Source: CAD feature listing. Evaluate the final solid. Frame: model axes, mm. Round coordinates to 2 decimals unless told otherwise and drop trailing zeros. Loops run counter-clockwise (first coordinate to the right, second up) from the corner with the lowest first, then second, coordinate; pieces in that order, holes last. Notation, with made-up numbers: M 41,27.5 L 73,27.5 A11 ccw 73,31.5 Z; hole C -1,73 d9. An arc over 180 degrees is marked long. One line per item, written item: value.
from build123d import *

# Parameters (mm, degrees)
SKETCH1_W                = 270
SKETCH1_H                = 25
BOSS_EXTRUDE1_DEPTH      = 4
M5_CLEARANCE_SLOT1_DEPTH = 4
LPATTERN1_COUNT          = 4
LPATTERN1_PITCH          = 82
M3_TAPPED_HOLE1_D        = 2.5
LPATTERN2_COUNT          = 8
LPATTERN2_PITCH          = 35.714285714
CHAMFER1_SIZE            = 2
M5_TAPPED_HOLE1_D        = 4.2


# Read off the part's stored shape, not the designer's step: M5 Clearance Slot1
with BuildPart() as part:
    # Sketch1 → Boss-Extrude1 (new body)
    with BuildSketch(Plane.XY):
        Rectangle(SKETCH1_W, SKETCH1_H)
    extrude(amount=BOSS_EXTRUDE1_DEPTH)

    # M5 Clearance Slot1 outline → M5 Clearance Slot1 (cut)
    with BuildSketch(Plane.XY):
        with BuildLine():
            Line((-120.25, 2.25), (-120.25, 6.75))
            ThreePointArc((-120.25, 6.75), (-123, 9.5), (-125.75, 6.75))
            Line((-125.75, 6.75), (-125.75, 2.25))
            ThreePointArc((-125.75, 2.25), (-123, -0.5), (-120.25, 2.25))
        make_face()
    m5_clearance_slot1 = extrude(amount=M5_CLEARANCE_SLOT1_DEPTH, mode=Mode.SUBTRACT)

    # LPattern1: M5 Clearance Slot1 ×4
    with Locations(*[(i * LPATTERN1_PITCH, 0, 0) for i in range(1, LPATTERN1_COUNT)]):
        add(m5_clearance_slot1, mode=Mode.SUBTRACT)

    # M3 Tapped Hole1 (through all)
    with Locations(Plane.XY.offset(4)):
        with Locations((-125, -7.5)):
            m3_tapped_hole1 = Hole(M3_TAPPED_HOLE1_D / 2)

    # LPattern2: M3 Tapped Hole1 ×8
    with Locations(*[(i * LPATTERN2_PITCH, 0, 0) for i in range(1, LPATTERN2_COUNT)]):
        add(m3_tapped_hole1, mode=Mode.SUBTRACT)

    # Chamfer1
    chamfer1_edges = [part.edges().sort_by_distance(p)[0] for p in [
        (-135, 12.5, 2),
        (135, 12.5, 2),
        (135, -12.5, 2),
        (-135, -12.5, 2),
    ]]
    chamfer(chamfer1_edges, length=CHAMFER1_SIZE)

    # M5 Tapped Hole1 (through all)
    with Locations(Plane.XY.offset(4)):
        with Locations((82, 4.5), (-82, 4.5)):
            Hole(M5_TAPPED_HOLE1_D / 2)


solid = part.part
1. Ray query, line 1 (Y direction, x = -82, z = 3); line 2 (X direction, y = 0.75, z = 0.9); line 3 (Y direction, x = -125, z = 2). Return the intervals inside material, ascending. Write a range as [from, to].
Report:
line 1: y = [-12.5, 2.4], [6.6, 12.5]
line 2: x = [-135, -125.3], [-120.7, -43.3], [-38.7, 38.7], [43.3, 120.7], [125.3, 135]
line 3: y = [-12.5, -8.75], [-6.25, 0.36], [8.64, 12.5]
2. Section query A-A (x = 41). Return the cut outline in (y, z), and give its area (3 significant figures).
Report:
outline: M -12.5,0 L -0.5,0 L -0.5,4 L -12.5,4 Z; M 9.5,0 L 12.5,0 L 12.5,4 L 9.5,4 Z
area: 60.0 mm2
3. Section query B-B (z = 1.1). Count the separate pieces of the cut face and the enclosed holes in it, and give its area (3 significant figures).
Report:
separate pieces: 1
enclosed holes: 14
area: 6,480 mm2
4. Pull-direction query (X, two-part tool) for faces 1 (the face through (-2, 0, 0)), 2 (the face through (84.1, 4.59, 1.97)); classes: released by +X, released by -X, zero draft, split by the parting line, or undercut.
Report:
face 1: zero draft
face 2: undercut
5. Pin query (flat end, axial travel): pin 1 (3 mm diameter, centred on x = 53.57, y = -7.5, fed in from +Z); pin 2 (2.5 mm diameter, centred on x = -82, y = 4.5, fed in from -Z). Return the tip coordinate at first contact, or that it passes through.
Report:
pin 1: stops at z = 4
pin 2: passes through
